The model under review builds one solid part; all positions refer to its coordinate system, in mm. A direction names the side the tool comes from. Round coordinates to 2 decimals unless told otherwise and drop trailing zeros. Write each loop counter-clockwise with the first axis right and the second up, starting at its lowest first coordinate (ties: lowest second). Pieces come first, ordered by that corner, then holes. Notation, with made-up numbers: (6, 28) -> (61, 28) arc R10 ccw to (61, 46) -> close; hole circle Ø7 at (48, 64.5). An arc over 180 degrees is marked (long way). Return JSON: item names as keys, results as strings. Group by question number.
1. Clearance check with flat-ended pins moving along their axes: P1, Ø7.5, axis at y = 10.5, z = 29, coming from the -X side; P2, Ø3, axis at y = 25, z = 19, coming from the +X side; P3, Ø1, axis at x = 59, y = 6.5, coming from the -Z side. State where each tip first meets the part, or that it passes through.
2. Take a section at C-C, the plane x = -58. Write out the cut boundary in (y, z).
3. Tool access review of faces 1 (the flat face through (-85, -6, 16.71)), 2 (the flat face through (73.011, 11, 29)), 3 (the flat face through (-1, -6, -59.49)): name each direction out of +Z, -Z, +X, -X, +Y, -Y from which nothing blocks a thin tool from reaching the whole face with its end or side.
4. Take a section at B-B, the plane y = -4. Write out the cut boundary in (x, z), then the cut area to 3 significant figures.
5. Take a section at A-A, the plane x = 0. Write out the cut boundary in (y, z).
6. Mouldability with a two-part tool opening along X and no side actions: class faces 4 (the cylindrical face through (81.487, -6.261, -3.85)), 5 (the flat face through (-1, 0, -38)), 6 (the cylindrical face through (-2.335, -6.261, -1.267)) as pulls with the +X half, pulls with the -X half, needs draft (parallel to the pull), parting line crosses it, or undercut.
7. Take a section at D-D, the plane z = -34. Write out the cut boundary in (x, y).
8. For line 1 along Z through (x, y) = (0, -5); line 2 along Y through (x, z) = (-43, -2.5); line 3 along Z through (x, y) = (19, 24), list the stretches that pass through material, from the lowest coordinate up. Write a range as from..to.
from build123d import *

# Parameters (mm, degrees)
F0_R     = 17.937476
F1_DEPTH = 12.7
F2_W     = 150.962264
F2_H     = 47.064063
F3_DEPTH = 25.4


with BuildPart() as f1:
    # F0 (on Front) → F1 (new body)
    with BuildSketch(Plane.XZ):
        with BuildLine():
            Line((72.837895, 16.709986), (-101.6, 16.709986))
            Line((-101.6, 16.709986), (-101.6, -59.490014))
            Line((-101.6, -59.490014), (101.6, -59.490014))
            Line((101.6, -59.490014), (101.6, -12.052119))
            ThreePointArc((101.6, -12.052119), (81.26212, -3.627894), (72.837895, 16.709986))
        make_face()
        with Locations((0, -19.051408)):
            Circle(F0_R, mode=Mode.SUBTRACT)
    extrude(amount=F1_DEPTH)

    # F2 (on face) → F3 (join)
    with BuildSketch(Plane.XY.offset(16.709986)):
        with Locations((-2.470292, 10.832032)):
            Rectangle(F2_W, F2_H)
    extrude(amount=F3_DEPTH)


solid = f1.part
Output:
{
 "1": {"P1": "stops at x = -77.95", "P2": "stops at x = 73.01", "P3": "stops at z = 16.71"},
 "2": {"outline": "(-12.7, -59.49) -> (0, -59.49) -> (0, 16.71) -> (34.36, 16.71) -> (34.36, 42.11) -> (-12.7, 42.11) -> close"},
 "3": {"face 1": "+Z, -X, +Y, -Y", "face 2": "+Z, +X, +Y, -Y", "face 3": "-Z, +X, -X, +Y, -Y"},
 "4": {"outline": "(-101.6, -59.49) -> (101.6, -59.49) -> (101.6, -12.05) arc R28.76 cw to (72.84, 16.71) -> (73.01, 16.71) -> (73.01, 42.11) -> (-77.95, 42.11) -> (-77.95, 16.71) -> (-101.6, 16.71) -> close; hole circle Ø35.87 at (0, -19.05)", "area": "17,700 mm^2"},
 "5": {"outline": "(-12.7, -59.49) -> (0, -59.49) -> (0, -36.99) -> (-12.7, -36.99) -> close; (-12.7, -1.11) -> (0, -1.11) -> (0, 16.71) -> (34.36, 16.71) -> (34.36, 42.11) -> (-12.7, 42.11) -> close"},
 "6": {"face 4": "pulls with the +X half", "face 5": "needs draft", "face 6": "undercut"},
 "7": {"outline": "(-101.6, -12.7) -> (-9.91, -12.7) -> (-9.91, 0) -> (-101.6, 0) -> close; (9.91, -12.7) -> (101.6, -12.7) -> (101.6, 0) -> (9.91, 0) -> close"},
 "8": {"line 1": "z = -59.49..-36.99, -1.11..42.11", "line 2": "y = -12.7..0", "line 3": "z = 16.71..42.11"}
}
